```python
from build123d import *

# Parameters (mm, degrees)
PAD_DEPTH    = 10
POCKET_DEPTH = 10.001
FILLET_R     = 1


with BuildPart() as part:
    # Sketch → Pad (new body)
    with BuildSketch(Plane.XY):
        with BuildLine():
            ThreePointArc((-7.064283, 4.064283), (0, -8.15), (7.064283, 4.064283))
            Line((10, 7), (7.064283, 4.064283))
            Line((10, 8.8), (10, 7))
            Line((2.7, 8.8), (10, 8.8))
            Line((2.7, 12), (2.7, 8.8))
            Line((5, 12), (2.7, 12))
            Line((3, 15), (5, 12))
            Line((-3, 15), (3, 15))
            Line((-5, 12), (-3, 15))
            Line((-2.7, 12), (-5, 12))
            Line((-2.7, 8.8), (-2.7, 12))
            Line((-10, 8.8), (-2.7, 8.8))
            Line((-10, 7), (-10, 8.8))
            Line((-7.064283, 4.064283), (-10, 7))
        make_face()
    extrude(amount=PAD_DEPTH)

    # Sketch001 → Pocket (cut, through all)
    with BuildSketch(Plane.XY.offset(10)):
        with BuildLine():
            ThreePointArc((2.4, -4.156922), (0, 4.8), (-2.4, -4.156922))
            Line((-2.4, -4.156922), (-2.614108, -9.156922))
            Line((-2.614108, -9.156922), (2.614108, -9.156922))
            Line((2.614108, -9.156922), (2.4, -4.156922))
        make_face()
    extrude(amount=-POCKET_DEPTH, mode=Mode.SUBTRACT)

    # Fillet
    fillet_edges = [part.edges().sort_by_distance(p)[0] for p in [
        (-2.553419, -7.739674, 5),
        (2.553419, -7.739674, 5),
    ]]
    fillet(fillet_edges, radius=FILLET_R)


solid = part.part
```
The listing builds one solid part. Answer for the finished solid, in the listing's coordinates (mm). A direction names the side the tool comes from. Give positions to 0.01 mm unless a question says otherwise; leave off trailing zeros. Order: outer loops, then holes, each group sorted by start corner. A loop starts at its lowest first (then second) coordinate and runs counter-clockwise, first axis right, second up. Notation, with made-up numbers: (85, 34) -> (94, 34) arc R15 cw to (94, 47) -> close; hole circle Ø8 at (-8.75, -38.75). An arc over 180 degrees is marked (long way). Answer as a JSON object with one key per item and string values. Group by question number.
Item 1: Flat-ended cylindrical pins translate along their axes: pin 1 (2 mm diameter, centred on x = 8, z = 6.5, fed in from +Y); pin 2 (2.5 mm diameter, centred on y = 10.5, z = 6.5, fed in from -X); pin 3 (1.5 mm diameter, centred on y = -5, z = 1.5, fed in from -X). Find the tip coordinate at first contact, or state that the pin passes through.
Item 2: The part is cut by section C-C on z = 7.75. Write down the section's boundary in (x, y).
Item 3: A tool of negligible diameter and unlimited length cuts with its end or side. For faces 1 (the flat face through (0, 15, 5)), 2 (the flat face through (-2.445, -5.205, 5.07)), 3 (the flat face through (6, 8.8, 5)), 4 (the flat face through (-6, 8.8, 5)), 5 (the flat face through (10, 8, 5)), from which of +Z, -Z, +X, -X, +Y, -Y can it reach the whole face along a straight path? Write none if from no direction.
Item 4: The part is cut by section B-B on x = -7.5. Write down the section's boundary in (y, z).
Item 5: The part is cut by section A-A on y = 0. Write down the section's boundary in (x, z).
Item 6: The part is cut by section D-D on x = 0. Write down the section's boundary in (y, z), and give its area (3 significant figures).
Item 7: Determine the mould class of faces 6 (the flat face through (9, 6, 5)), 7 (the cylindrical face through (-7.88, -2.08, 4.93)), 8 (the cylindrical face through (3.015, -7.12, 4.93)), 9 (the flat face through (4, 12, 5)) for opening direction X: pulls with the +X half, pulls with the -X half, needs draft (parallel to the pull), parting line crosses it, or undercut.
Item 8: Consider L1, parallel to X at y = 0, z = 4; L2, parallel to Y at x = 0, z = 7; L3, parallel to X at y = -5.75, z = 8. Determine where each line is inside the solid, lowest interval first. Write a range as from..to.
Result set:
{
 "1": {"pin 1": "y = 8.8", "pin 2": "x = -2.7", "pin 3": "x = -6.95"},
 "2": {"outline": "(-10, 7) -> (-7.06, 4.06) arc R8.15 ccw to (-3.98, -7.11) arc R1 ccw to (-2.49, -6.28) -> (-2.4, -4.16) arc R4.8 cw (long way) to (2.4, -4.16) -> (2.49, -6.28) arc R1 ccw to (3.98, -7.11) arc R8.15 ccw to (7.06, 4.06) -> (10, 7) -> (10, 8.8) -> (2.7, 8.8) -> (2.7, 12) -> (5, 12) -> (3, 15) -> (-3, 15) -> (-5, 12) -> (-2.7, 12) -> (-2.7, 8.8) -> (-10, 8.8) -> close"},
 "3": {"face 1": "+Z, -Z, +X, -X, +Y", "face 2": "+Z, -Z, -Y", "face 3": "+Z, -Z, +X", "face 4": "+Z, -Z, -X", "face 5": "+Z, -Z, +X, +Y, -Y"},
 "4": {"outline": "(-3.19, 0) -> (3.19, 0) -> (3.19, 10) -> (-3.19, 10) -> close; (4.5, 0) -> (8.8, 0) -> (8.8, 10) -> (4.5, 10) -> close"},
 "5": {"outline": "(-8.15, 0) -> (-4.8, 0) -> (-4.8, 10) -> (-8.15, 10) -> close; (4.8, 0) -> (8.15, 0) -> (8.15, 10) -> (4.8, 10) -> close"},
 "6": {"outline": "(4.8, 0) -> (15, 0) -> (15, 10) -> (4.8, 10) -> close", "area": "102 mm²"},
 "7": {"face 6": "pulls with the +X half", "face 7": "pulls with the -X half", "face 8": "undercut", "face 9": "needs draft"},
 "8": {"L1": "-8.15..-4.8, 4.8..8.15", "L2": "4.8..15", "L3": "-5.78..-2.47, 2.47..5.78"}
}
